from build123d import *

# Parameters (mm, degrees)
CROQUIS21_W             = 34
CROQUIS21_H             = 30
SALIENTE_EXTRUIR4_DEPTH = 17.5
CORTAR_EXTRUIR17_REACH  = 63.934
CROQUIS22_W             = 24
CROQUIS22_H             = 10
CORTAR_EXTRUIR18_REACH  = 50.603
CROQUIS23_W             = 11
CROQUIS23_H             = 15
CORTAR_EXTRUIR19_REACH  = 70.953
CROQUIS24_R             = 2.5
CROQUIS25_R             = 4.65
CORTAR_EXTRUIR20_DEPTH  = 2.5
REDONDEO2_R             = 10
REDONDEO3_R             = 5
CROQUIS27_R             = 2
SALIENTE_EXTRUIR5_DEPTH = 5
CROQUIS30_R             = 3.25
CORTAR_EXTRUIR21_DEPTH  = 2


# Some blends are built 0.0001 mm under size
with BuildPart() as part:
    # Croquis21 → Saliente-Extruir4 (new, symmetric)
    with BuildSketch(Plane(origin=(0, 0, 0), x_dir=(1, 0, 0), z_dir=(0, 1, 0))):
        with Locations((34.278993672, -15)):
            Rectangle(CROQUIS21_W, CROQUIS21_H)
    extrude(amount=SALIENTE_EXTRUIR4_DEPTH, both=True)

    # Croquis22 → Cortar-Extruir17 (cut, up to next)
    with BuildSketch(Plane.XY.offset(30), mode=Mode.PRIVATE) as cortar_extruir17_sk1:
        with Locations((34.278993672, 7.5)):
            Rectangle(CROQUIS22_W, CROQUIS22_H)
    cortar_extruir17_tool1 = extrude(cortar_extruir17_sk1.sketch, amount=-CORTAR_EXTRUIR17_REACH, mode=Mode.PRIVATE) & part.part
    # Croquis22 → Cortar-Extruir17 (cut, up to next)
    with BuildSketch(Plane.XY.offset(30), mode=Mode.PRIVATE) as cortar_extruir17_sk2:
        with Locations((34.278993672, -7.5)):
            Rectangle(CROQUIS22_W, CROQUIS22_H)
    cortar_extruir17_tool2 = extrude(cortar_extruir17_sk2.sketch, amount=-CORTAR_EXTRUIR17_REACH, mode=Mode.PRIVATE) & part.part
    add(cortar_extruir17_tool1.solids().sort_by_distance((34.278994, 7.5, 30))[0], mode=Mode.SUBTRACT)
    add(cortar_extruir17_tool2.solids().sort_by_distance((34.278994, -7.5, 30))[0], mode=Mode.SUBTRACT)

    # Croquis23 → Cortar-Extruir18 (cut, up to next)
    with BuildSketch(Plane.ZY.offset(-17.278993672), mode=Mode.PRIVATE) as cortar_extruir18_sk1:
        with Locations((5.5, 10)):
            Rectangle(CROQUIS23_W, CROQUIS23_H)
    cortar_extruir18_tool1 = extrude(cortar_extruir18_sk1.sketch, amount=-CORTAR_EXTRUIR18_REACH, mode=Mode.PRIVATE) & part.part
    add(cortar_extruir18_tool1.solids().sort_by_distance((17.278994, 10, 5.5))[0], mode=Mode.SUBTRACT)

    # Cortar-Extruir19: up to this face of the body (flat: up to its plane)
    cortar_extruir19_end = Plane(part.part.faces().sort_by_distance((34.278993672, -17.5, 15))[0])
    # Croquis24 → Cortar-Extruir19 (cut, up to the picked face)
    with BuildSketch(Plane(origin=(0, 17.5, 0), x_dir=(1, 0, 0), z_dir=(0, 1, 0)), mode=Mode.PRIVATE) as cortar_extruir19_sk1:
        with Locations(Location((34.278993672, -21, 0), (0, 0, 270))):
            Circle(CROQUIS24_R)
    cortar_extruir19_tool1 = split(extrude(cortar_extruir19_sk1.sketch, amount=-CORTAR_EXTRUIR19_REACH, mode=Mode.PRIVATE), bisect_by=cortar_extruir19_end, keep=Keep.BOTH, mode=Mode.PRIVATE)
    add(cortar_extruir19_tool1.solids().sort_by(Axis((34.278994, 17.5, 21), (0, -1, 0)))[0], mode=Mode.SUBTRACT)

    # Croquis25 → Cortar-Extruir20 (cut)
    with BuildSketch(Plane(origin=(0, 17.5, 0), x_dir=(1, 0, 0), z_dir=(0, 1, 0))):
        with Locations(Location((34.278993672, -21, 0), (0, 0, 270))):
            Circle(CROQUIS25_R)
    extrude(amount=-CORTAR_EXTRUIR20_DEPTH, mode=Mode.SUBTRACT)

    # Redondeo2
    # the kernel refuses this fillet: 10 mm, written as the material it takes off along each edge
    with BuildSketch(Plane(origin=(51.278993672, 42.5, 30), x_dir=(0, 0, -1), z_dir=(0, -1, 0)), Plane(origin=(17.278993672, -42.5, 30), x_dir=(0, 0, -1), z_dir=(0, 1, 0))) as redondeo2_piece_1:
        with BuildLine():
            CenterArc((REDONDEO2_R, -REDONDEO2_R), REDONDEO2_R, 90, 90)
            Line((0, -REDONDEO2_R), (0, 0))
            Line((0, 0), (REDONDEO2_R, 0))
        make_face()
    extrude(amount=85, mode=Mode.SUBTRACT)

    # Redondeo3
    redondeo3_edges = [part.edges().sort_by_distance(p)[0] for p in [
        (46.278993672, 12.5, 19.830127019),
        (46.278993672, 2.5, 19.830127019),
        (46.278993672, -12.5, 14.330127019),
        (22.278993672, -12.5, 14.330127019),
        (22.278993672, -2.5, 14.330127019),
        (22.278993672, 12.5, 19.830127019),
        (22.278993672, 2.5, 19.830127019),
        (46.278993672, -2.5, 14.330127019),
    ]]
    fillet(redondeo3_edges, radius=REDONDEO3_R - 0.0001)  # a hair under: the kernel refuses the full size

    # Croquis27 → Saliente-Extruir5 (add)
    # profile 1 of 2: a face of its own
    with BuildSketch(Plane(origin=(0, -12.5, 0), x_dir=(1, 0, 0), z_dir=(0, 1, 0))):
        with BuildLine():
            Line((27.278993672, -30), (17.278993672, -30))
            Line((17.278993672, -30), (-7.721006328, -30))
            Line((-7.721006328, -30), (-7.721006328, 0))
            Line((-7.721006328, 0), (17.278993672, 0))
            Line((17.278993672, 0), (17.278993672, -20))
            ThreePointArc((17.278993672, -20), (20.20792586, -27.071067812), (27.278993672, -30))
        make_face()
        with Locations(Location((-2.721006328, -6, 0), (0, 0, 270))):
            Circle(CROQUIS27_R, mode=Mode.SUBTRACT)
        with Locations(Location((-2.721006328, -24, 0), (0, 0, 90))):
            Circle(CROQUIS27_R, mode=Mode.SUBTRACT)
    # profile 2 of 2: a face of its own
    with BuildSketch(Plane(origin=(0, -12.5, 0), x_dir=(1, 0, 0), z_dir=(0, 1, 0))):
        with BuildLine():
            Line((51.278993672, 0), (51.278993672, -20))
            ThreePointArc((51.278993672, -20), (48.350061484, -27.071067812), (41.278993672, -30))
            Line((41.278993672, -30), (61.278993672, -30))
            Line((61.278993672, -30), (61.278993672, 0))
            Line((61.278993672, 0), (51.278993672, 0))
        make_face()
        with Locations(Location((56.278993672, -6, 0), (0, 0, 90))):
            Circle(CROQUIS27_R, mode=Mode.SUBTRACT)
        with Locations(Location((56.278993672, -24, 0), (0, 0, 270))):
            Circle(CROQUIS27_R, mode=Mode.SUBTRACT)
    extrude(amount=-SALIENTE_EXTRUIR5_DEPTH)

    # Croquis30 → Cortar-Extruir21 (cut)
    with BuildSketch(Plane(origin=(0, -12.5, 0), x_dir=(1, 0, 0), z_dir=(0, 1, 0))):
        with Locations(Location((-2.721006328, -6, 0), (0, 0, 270))):
            Circle(CROQUIS30_R)
        with Locations(Location((-2.721006328, -24, 0), (0, 0, 90))):
            Circle(CROQUIS30_R)
        with Locations(Location((56.278993672, -6, 0), (0, 0, 90))):
            Circle(CROQUIS30_R)
        with Locations(Location((56.278993672, -24, 0), (0, 0, 270))):
            Circle(CROQUIS30_R)
        Polygon((3.278993672, -4.5), (14.278993672, -4.5), (14.278993672, -9.5), (14.278993672, -20.5), (14.278993672, -25.5), (3.278993672, -25.5), (3.278993672, -20.5), (-6.721006328, -20.5), (-6.721006328, -9.5), (3.278993672, -9.5), align=None)
    extrude(amount=-CORTAR_EXTRUIR21_DEPTH, mode=Mode.SUBTRACT)


solid = part.part
Work out the finished part from the listing and answer in its coordinate system (mm). A direction names the side the tool comes from. Give positions to 0.01 mm unless a question says otherwise; leave off trailing zeros. Write each loop counter-clockwise with the first axis right and the second up, starting at its lowest first coordinate (ties: lowest second). Pieces come first, ordered by that corner, then holes.
Q1. The part is cut by section B-B on y = -10. Give the vertices of the cut face in (x, z), and give its area (3 significant figures).
Answer:
outline: (17.28, 0) - (22.95, 0) - (22.95, 29.01) arc R10 ccw to (17.28, 20) - close; (45.61, 0) - (51.28, 0) - (51.28, 20) arc R10 ccw to (45.61, 29.01) - close
area: 300 mm2
Q2. The part is cut by section C-C on x = 55.5. Give the vertices of the cut face in (y, z).
Answer:
outline: (-17.5, 0) - (-12.5, 0) - (-12.5, 2.84) - (-14.5, 2.84) - (-14.5, 4.16) - (-17.5, 4.16) - close; (-17.5, 7.84) - (-14.5, 7.84) - (-14.5, 9.16) - (-12.5, 9.16) - (-12.5, 20.84) - (-14.5, 20.84) - (-14.5, 22.16) - (-17.5, 22.16) - close; (-17.5, 25.84) - (-14.5, 25.84) - (-14.5, 27.16) - (-12.5, 27.16) - (-12.5, 30) - (-17.5, 30) - close
Q3. The part is cut by section D-D on z = 17.5. State how many separate pieces and enclosed holes the cut face has, and give its area (3 significant figures).
Answer:
separate pieces: 1
enclosed holes: 2
area: 871 mm2
Q4. A tool of negligible diameter and unlimited length cuts with its end or side. For faces 1 (the face through (-2, -13, 20.5)), 2 (the face through (23.705, -4.004, 14.79)), 3 (the face through (58.053, -15.979, 5.077)), 4 (the face through (34, 13, 11)), from which of +Z, -Z, +X, -X, +Y, -Y can it reach the whole face along a straight path? Write none if from no direction.
Answer:
face 1: +Y
face 2: +Z, -Z
face 3: +Y, -Y
face 4: -Z, +X, -X, +Y
Q5. Straight lines are drawn through the part: L1, parallel to Y at x = 34.5, z = 13; L2, parallel to X at y = -15.8, z = 24; L3, parallel to Y at x = 27, z = 3. For each, find the intervals that lie inside material, in ascending order.
Answer:
L1: y = -17.5 to -12.5, -2.5 to 2.5, 12.5 to 17.5
L2: x = -7.72 to -4.72, -0.72 to 54.28, 58.28 to 61.28
L3: y = -17.5 to -12.49, -2.51 to 2.5
Q6. Given pin 1 (2 mm diameter, centred on x = 52, z = 3.5, fed in from +Y); pin 2 (7 mm diameter, centred on x = 56.5, z = 24, fed in from +Y); pin 3 (8.5 mm diameter, centred on x = 56.28, z = 24, fed in from -Y); pin 4 (6.5 mm diameter, centred on x = 34.28, z = 21, fed in from +Y), each flat-ended and moving along its own axis, determine where each tip first touches the part or whether it passes through.
Answer:
pin 1: stops at y = 2.5
pin 2: stops at y = -12.5
pin 3: stops at y = -17.5
pin 4: stops at y = 15
Q7. For a pull along X with two mould halves and no side action, classify faces 5 (the face through (-6.721, -13, 15)), 6 (the face through (34, 0, 30)), 7 (the face through (32.6, 12.5, 18.5)) as released by +X, released by -X, zero draft, split by the parting line, or undercut.
Answer:
face 5: undercut
face 6: zero draft
face 7: undercut
Q8. The part is cut by section A-A on x = 11. Give the vertices of the cut face in (y, z).
Answer:
outline: (-17.5, 0) - (-12.5, 0) - (-12.5, 4.5) - (-14.5, 4.5) - (-14.5, 25.5) - (-12.5, 25.5) - (-12.5, 30) - (-17.5, 30) - close
